```python
from build123d import *

# Parameters (mm, degrees)
F2_R     = 1.75
F3_SIZE  = 1
F4_R     = 4
F5_DEPTH = 25
F6_SIZE  = 0.5
F7_SIZE  = 0.5


with BuildPart() as f1:
    # F0 (on Front) → F1 (revolve)
    with BuildSketch(Plane.XZ):
        with BuildLine():
            Line((0, 36.387), (0, 25))
            Line((0, 25), (3, 20.715556))
            Line((3, 20.715556), (3, 7))
            Line((3, 7), (6.5, 7))
            Line((6.5, 7), (6.5, 9))
            Line((6.5, 9), (12, 9))
            Line((12, 9), (12, 17.5))
            Line((12, 17.5), (6, 17.5))
            Line((6, 17.5), (6, 36.387))
            Line((6, 36.387), (5.078729, 38.611145))
            ThreePointArc((5.078729, 38.611145), (3, 40.000107), (0.921271, 38.611145))
            Line((0.921271, 38.611145), (0, 36.387))
        make_face()
    revolve(axis=Axis((11.340396, 0, 0), (1, 0, 0)))

    # F2
    f2_edges = [f1.edges().sort_by_distance(p)[0] for p in [
        (6, 0, -17.5),
    ]]
    fillet(f2_edges, radius=F2_R)

    # F3
    f3_edges = [f1.edges().sort_by_distance(p)[0] for p in [
        (12, 0, -17.5),
    ]]
    chamfer(f3_edges, length=F3_SIZE)

    # F4 (on face) → F5 (cut)
    with BuildSketch(Plane(origin=(0, 0, 0), x_dir=(0, -1, 0), z_dir=(-1, 0, 0))):
        with Locations((0, 31)):
            Circle(F4_R)
        with Locations((-26.846788, -15.5)):
            Circle(F4_R)
        with Locations((26.846788, -15.5)):
            Circle(F4_R)
    extrude(amount=-F5_DEPTH, mode=Mode.SUBTRACT)

    # F6
    f6_edges = [f1.edges().sort_by_distance(p)[0] for p in [
        (6.5, 0, -7),
    ]]
    chamfer(f6_edges, length=F6_SIZE)

    # F7
    f7_edges = [f1.edges().sort_by_distance(p)[0] for p in [
        (3, 0, -7),
    ]]
    chamfer(f7_edges, length=F7_SIZE)


solid = f1.part
```
For this review, take the finished solid that the model builds, in its own axes (mm). A direction names the side the tool comes from. Round coordinates to 2 decimals unless told otherwise and drop trailing zeros.
Q1. Insertion check: pin 1 Ø8.5 at (y, z) = (0, 0) entering from +X; pin 2 Ø10.5 at (y, z) = (26.85, -15.5) entering from +X; pin 3 Ø1.5 at (x, z) = (4, -27.5) entering from -Y; pin 4 Ø5 at (x, y) = (5.5, -19.5) entering from +Z. Each pin has a flat end and moves straight along its axis. Give the tip position at first contact, or say it passes through.
Result sheet:
pin 1: passes through
pin 2: stops at x = 6
pin 3: stops at y = -29.53
pin 4: stops at z = 35.72
Q2. Mouldability with a two-part tool opening along Y and no side actions: class faces 4 (the face through (5.94, 35.66, -7.92)), 5 (the face through (12, 7, -7)), 6 (the face through (2.85, -20.75, -2.72)) as +Y half, -Y half, draft (parallel to the pull), parting line (faces both ways), or undercut.
Result sheet:
face 4: parting line
face 5: draft
face 6: undercut
Q3. Machinability: for faces 1 (the face through (3, 9, 0)), 2 (the face through (6, 16, -16)), 3 (the face through (4.768, 2.681, 6.466)), which of the approach directions +Z, -Z, +X, -X, +Y, -Y give a long, thin tool a straight path to every point of the face, cutting with its end or side? Answer none if there is none.
Result sheet:
face 1: -X
face 2: +X
face 3: +X, -X
Q4. Add section B-B on y = 0. Give the number of separate pieces and of enclosed holes in the cut face, plus the area to 3 significant figures.
Result sheet:
separate pieces: 3
enclosed holes: 0
area: 344 mm2
Q5. To check wall thickness, follow line 1 along Z through (x, y) = (10, 0); line 2 along X through (y, z) = (6.5, 30.5); line 3 along X through (y, z) = (-16, 7.5). State the ranges of each line that lie inside material, in increasing order.
Result sheet:
line 1: z = -17.5 to -9, 9 to 17.5
line 2: x = 0 to 6
line 3: x = 3 to 7
